CAD build for the part. Positions are in the model's coordinates, mm. Give positions to 0.01 mm unless a question says otherwise; leave off trailing zeros. Write each loop counter-clockwise with the first axis right and the second up, starting at its lowest first coordinate (ties: lowest second). Pieces come first, ordered by that corner, then holes. Notation, with made-up numbers: (-21.75, 63) - (15.25, 63) arc R36 ccw to (15.25, 99) - close; hole circle Ø1 at (41, 73.25). An arc over 180 degrees is marked (long way). Put each result on its own line as item: value. Start each with the question number.
1. Cut at C-C on x = 10. List the corners of the cut face in (y, z).
2. Cut at A-A on y = -4.5. List the corners of the cut face in (x, z).
3. Wall check: line 1 (X direction, y = 9.5, z = 0.2); line 2 (Y direction, x = 13.5, z = 0.6); line 3 (X direction, y = 14, z = 2.2). Give the ranges that are in metal, low to high.
4. Cut at B-B on z = 0.65. List the corners of the cut face in (x, y) (3 decimals), and give its area (3 significant figures).
5. Cut at D-D on x = 1. List the corners of the cut face in (y, z), and give its area (3 significant figures).
6. Drop flat-ended pins along their axis: pin 1 (8 mm diameter, centred on x = 3, y = 10.5, fed in from -Z); pin 2 (1 mm diameter, centred on x = -2.5, z = 1.5, fed in from -Y). Give the stop position or say it passes through.
from build123d import *

# Parameters (mm, degrees)
F1_DEPTH = 2.54


with BuildPart() as f1:
    # F0 (on Top) → F1 (new body)
    with BuildSketch(Plane.XY):
        with BuildLine():
            Line((19.939, 16.51), (-19.939, 16.51))
            Line((-19.939, 16.51), (-19.939, -16.51))
            Line((-19.939, -16.51), (-3.048, -16.51))
            Line((-3.048, -16.51), (-3.048, -12.7))
            Line((-3.048, -12.7), (-8.001, -12.7))
            ThreePointArc((-8.001, -12.7), (-9.525, -14.224), (-11.049, -12.7))
            Line((-11.049, -12.7), (-16.129, -12.7))
            Line((-16.129, -12.7), (-16.129, 12.7))
            Line((-16.129, 12.7), (-11.049, 12.7))
            ThreePointArc((-11.049, 12.7), (-9.525, 14.224), (-8.001, 12.7))
            Line((-8.001, 12.7), (8.001, 12.7))
            ThreePointArc((8.001, 12.7), (9.525, 14.224), (11.049, 12.7))
            Line((11.049, 12.7), (16.129, 12.7))
            Line((16.129, 12.7), (16.129, -12.7))
            Line((16.129, -12.7), (11.049, -12.7))
            ThreePointArc((11.049, -12.7), (9.525, -14.224), (8.001, -12.7))
            Line((8.001, -12.7), (3.048, -12.7))
            Line((3.048, -12.7), (3.048, -16.51))
            Line((3.048, -16.51), (19.939, -16.51))
            Line((19.939, -16.51), (19.939, 16.51))
        make_face()
    extrude(amount=F1_DEPTH)


solid = f1.part
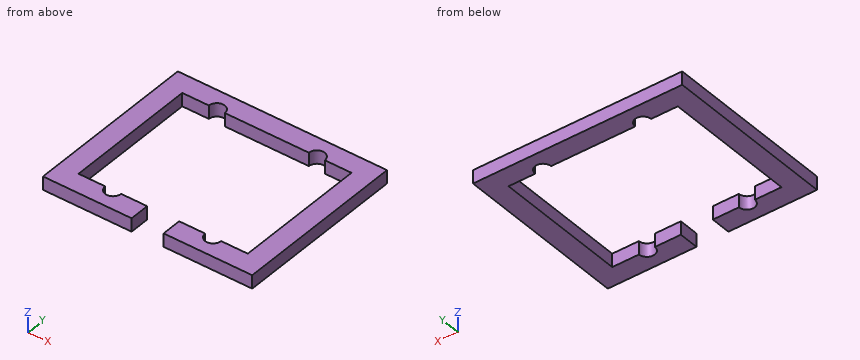
Report:
1. outline: (-16.51, 0) - (-14.15, 0) - (-14.15, 2.54) - (-16.51, 2.54) - close; (14.15, 0) - (16.51, 0) - (16.51, 2.54) - (14.15, 2.54) - close
2. outline: (-19.94, 0) - (-16.13, 0) - (-16.13, 2.54) - (-19.94, 2.54) - close; (16.13, 0) - (19.94, 0) - (19.94, 2.54) - (16.13, 2.54) - close
3. line 1: x = -19.94 to -16.13, 16.13 to 19.94
3. line 2: y = -16.51 to -12.7, 12.7 to 16.51
3. line 3: x = -19.94 to -10.32, -8.73 to 8.73, 10.32 to 19.94
4. outline: (-19.939, -16.51) - (-3.048, -16.51) - (-3.048, -12.7) - (-8.001, -12.7) arc R1.524 cw to (-11.049, -12.7) - (-16.129, -12.7) - (-16.129, 12.7) - (-11.049, 12.7) arc R1.524 cw to (-8.001, 12.7) - (8.001, 12.7) arc R1.524 cw to (11.049, 12.7) - (16.129, 12.7) - (16.129, -12.7) - (11.049, -12.7) arc R1.524 cw to (8.001, -12.7) - (3.048, -12.7) - (3.048, -16.51) - (19.939, -16.51) - (19.939, 16.51) - (-19.939, 16.51) - close
4. area: 460 mm²
5. outline: (12.7, 0) - (16.51, 0) - (16.51, 2.54) - (12.7, 2.54) - close
5. area: 9.68 mm²
6. pin 1: stops at z = 0
6. pin 2: stops at y = 12.7
